Read the model definition and answer for the solid it produces. Units are mm, in the model's axes. A direction names the side the tool comes from. Coordinates: 2 decimals unless noted, no trailing zeros. Write each loop counter-clockwise with the first axis right and the second up, starting at its lowest first coordinate (ties: lowest second). Pieces come first, ordered by that corner, then holes. Notation, with made-up numbers: (-34, 17) -> (-1, 17) arc R31 cw to (-1, 42) -> close; hole circle Ø7 at (33.25, -36.75). An arc over 180 degrees is marked (long way). Answer as a JSON object with one key per item and string values. Group by question number.
(1) Straight lines are drawn through the part: L1, parallel to Z at x = 7, y = 0.8 (3 decimals); L2, parallel to X at y = 1, z = 5 (3 decimals). For each, find the intervals that lie inside material, in ascending order.
(2) Find section C-C (z = 5). Give the vertices of the cut face in (x, y) (3 decimals), then the cut area to 3 significant figures.
(3) Which of the six approach directions +Z, -Z, +X, -X, +Y, -Y give full straight-line access (tool end or side, diameter ignored) to faces 5 (the face through (1, 10, 5)), 6 (the face through (2, 7, 5))?
(4) Find section D-D (x = 1.5). Give the vertices of the cut face in (y, z) (3 decimals), then the cut area to 3 significant figures.
(5) For a pull along Z with two mould halves and no side action, classify faces 1 (the face through (3.2, 1.7, 10)), 2 (the face through (9, 2, 5)), 3 (the face through (7.731, 1.014, 6.406)), 4 (the face through (1.014, 4.393, 3.536)) as +Z half, -Z half, draft (parallel to the pull), parting line (faces both ways), or undercut.
(6) Find section A-A (y = 5). Give the vertices of the cut face in (x, z) (3 decimals), then the cut area to 3 significant figures.
from build123d import *

# Parameters (mm, degrees)
BOSS_EXTRUDE1_DEPTH = 10
SKETCH2_R           = 1.585
CUT_EXTRUDE1_DEPTH  = 3
SKETCH3_R           = 1.585
CUT_EXTRUDE2_DEPTH  = 3


with BuildPart() as part:
    # Sketch1 → Boss-Extrude1 (new body)
    with BuildSketch(Plane.XY):
        Polygon((0, 0), (12, 0), (12, 2), (2, 2), (2, 10), (0, 10), align=None)
    extrude(amount=BOSS_EXTRUDE1_DEPTH)

    # Sketch2 → Cut-Extrude1 (cut, through all)
    with BuildSketch(Plane(origin=(0, 2, 0), x_dir=(1, 0, 0), z_dir=(0, 1, 0))):
        with Locations((7, -5)):
            Circle(SKETCH2_R)
    extrude(amount=-CUT_EXTRUDE1_DEPTH, mode=Mode.SUBTRACT)

    # Sketch3 → Cut-Extrude2 (cut, through all)
    with BuildSketch(Plane(origin=(2, 0, 0), x_dir=(0, 0, -1), z_dir=(1, 0, 0))):
        with Locations((-5, 5)):
            Circle(SKETCH3_R)
    extrude(amount=-CUT_EXTRUDE2_DEPTH, mode=Mode.SUBTRACT)


solid = part.part
Results below:
{
 "1": {"L1": "z = 0 to 3.415, 6.585 to 10", "L2": "x = 0 to 5.415, 8.585 to 12"},
 "2": {"outline": "(0, 0) -> (5.415, 0) -> (5.415, 2) -> (2, 2) -> (2, 3.415) -> (0, 3.415) -> close; (0, 6.585) -> (2, 6.585) -> (2, 10) -> (0, 10) -> close; (8.585, 0) -> (12, 0) -> (12, 2) -> (8.585, 2) -> close", "area": "27.3 mm2"},
 "3": {"face 5": "+Z, -Z, +X, -X, +Y", "face 6": "+Z, -Z, +X, +Y"},
 "4": {"outline": "(0, 0) -> (10, 0) -> (10, 10) -> (0, 10) -> close; hole circle Ø3.17 at (5, 5)", "area": "92.1 mm2"},
 "5": {"face 1": "+Z half", "face 2": "draft", "face 3": "undercut", "face 4": "undercut"},
 "6": {"outline": "(0, 0) -> (2, 0) -> (2, 3.415) -> (0, 3.415) -> close; (0, 6.585) -> (2, 6.585) -> (2, 10) -> (0, 10) -> close", "area": "13.7 mm2"}
}
